Design review of the part built by this model. Coordinates are the model's own, in mm. Face numbers are marked on the shaded views. A direction names the side the tool comes from. Coordinates: 2 decimals unless noted, no trailing zeros. Loops run counter-clockwise (first coordinate to the right, second up) from the corner with the lowest first, then second, coordinate; pieces in that order, holes last. Notation, with made-up numbers: (77, 81.25) - (97, 81.25) arc R28 ccw to (97, 99.25) - close; hole circle Ø1 at (49, -11.75). An arc over 180 degrees is marked (long way). Answer in a Markdown table with one row per item. Add a question column.
(1) To check wall thickness, follow L1, parallel to Y at x = 15.8, z = 35.05; L2, parallel to Y at x = 15, z = 34; L3, parallel to Z at x = -3.5, y = -14. State the ranges of each line that lie inside material, in increasing order. Write a range as [from, to].
(2) Clearance check with flat-ended pins moving along their axes: pin 1 (0.7 mm diameter, centred on y = -0.5, z = 49.5, fed in from -X); pin 2 (2.5 mm diameter, centred on x = -16, y = -15, fed in from +Z); pin 3 (1.5 mm diameter, centred on x = -15.5, y = 15.5, fed in from +Z). State where each tip first meets the part, or that it passes through.
(3) We need section C-C, the plane y = 15.8. Write out the cut boundary in (x, z).
(4) We need section A-A, the plane y = -12.5. Write out the cut boundary in (x, z), plus the area to 3 significant figures.
(5) For the marked faces 1 and 2, list the 3-axis set-ups (+Z, -Z, +X, -X, +Y, -Y) from which the entire face can be reached by the end or side of a thin tool; tool diameter is ignored.
(6) We need section B-B, the plane x = 0. Write out the cut boundary in (y, z), plus the area to 3 significant figures.
(7) The part is to be moulded in two halves that separate along X. For the marked faces 3, 4 and 5, say which applies: released by +X, released by -X, zero draft, split by the parting line, or undercut.
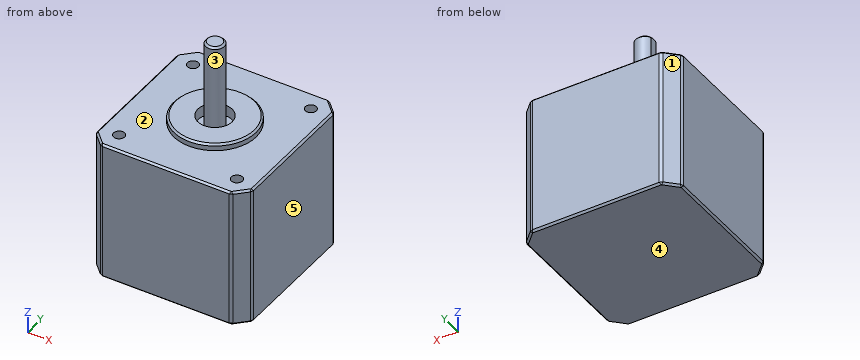
Autodesk Inventor part; units mm, degrees
ref_plane "YZ Plane" through (0, 0, 0) normal (1, 0, 0) x (0, 1, 0)
ref_plane "XZ Plane" through (0, 0, 0) normal (0, 1, 0) x (-1, 0, 0)
ref_plane "XY Plane" through (0, 0, 0) normal (0, 0, 1) x (1, 0, 0)
sketch "Sketch1" plane through (0, 0, 0) normal (0, 0, 1) x (1, 0, 0)
  line L0 (-17.4645, 21) -> (17.4645, 21)
  line L1 (21, 17.4645) -> (21, -17.4645)
  line L2 (17.4645, -21) -> (-17.4645, -21)
  line L3 (-21, -17.4645) -> (-21, 17.4645)
  line L4 (-21, 17.4645) -> (-17.4645, 21)
  line L5 (-21, 17.4645) -> (-16, 17.4645) construction
  line L6 (-17.4645, -21) -> (-21, -17.4645)
  line L7 (21, -17.4645) -> (17.4645, -21)
  line L8 (17.4645, 21) -> (21, 17.4645)
  point P0 (0, 0)
  point P1 (0, 21)
  point P2 (-21, 0)
  dimension "d4" = 360
  dimension "d1" = 45
  dimension "d6" = 5
  dimension "d7" = 42
  dimension "d8" = 42
extrude "Extrusion1" add sketch "Sketch1" along normal blind 37.5
sketch "Sketch2" plane through (0, 0, 37.5) normal (0, 0, 1) x (1, 0, 0)
  circle A0 centre (0, 0) radius 11
  dimension "d11" = 22
extrude "Extrusion2" add sketch "Sketch2" along normal blind 1.8
sketch "Sketch3" plane through (0, 0, 39.3) normal (0, 0, 1) x (1, 0, 0)
  circle A0 centre (0, 0) radius 4.6
  dimension "d14" = 9.2
extrude "Extrusion3" cut sketch "Sketch3" against normal blind 3
sketch "Sketch4" plane through (0, 0, 36.3) normal (0, 0, 1) x (1, 0, 0)
  circle A0 centre (0, 0) radius 2.5
  dimension "d17" = 5
extrude "Extrusion4" add sketch "Sketch4" along normal blind 24
sketch "Sketch5" plane through (0, 0, 60.3) normal (0, 0, 1) x (1, 0, 0)
  arc A0 (-2.25, 1.0897) -> (-2.25, -1.0897) centre (0, 0) ccw
  line L0 (-2.25, 1.0897) -> (-2.25, -1.0897)
  circle A1 centre (0, 0) radius 2.5
  dimension "d20" = 2.25
extrude "Extrusion5" cut sketch "Sketch5" against normal blind 21 contours L0 A0
chamfer "Chamfer1" distance 0.5 angle 45 2 edges at (0.559, -2.4367, 60.3) (0.559, 2.4367, 60.3)
sketch "Sketch6" plane through (0, 0, 37.5) normal (0, 0, 1) x (1, 0, 0)
  circle A0 centre (-15.8, 15.8) radius 1.5
  circle A1 centre (15.8, 15.8) radius 1.5
  circle A2 centre (-15.8, -15.8) radius 1.5
  circle A3 centre (15.8, -15.8) radius 1.5
  point P0 (0, 0)
  dimension "d27" = 15.8
  dimension "d28" = 31.6
  dimension "d29" = 15.8
  dimension "d30" = 31.6
  dimension "d31" = 3
extrude "Extrusion6" cut sketch "Sketch6" against normal blind 5
thread "Thread1"
thread "Thread2"
thread "Thread3"
thread "Thread4"
chamfer "Chamfer2" distance 0.5 angle 45 1 edges at (-11, 0, 39.3)
chamfer "Chamfer3" distance 0.5 angle 45 24 edges at (0, -21, 0) (19.2322, -19.2322, 0) (21, 0, 0) (-21, 0, 0) (0, 21, 0) (21, 0, 37.5) (0, 21, 37.5) (-21, 0, 37.5) (0, -21, 37.5) (19.2322, 19.2322, 37.5) (-19.2322, -19.2322, 37.5) (19.2322, -19.2322, 37.5) (17.4645, -21, 18.75) (21, -17.4645, 18.75) (-17.4645, -21, 18.75) (-21, -17.4645, 18.75) (21, 17.4645, 18.75) (17.4645, 21, 18.75) (-17.4645, 21, 18.75) (-21, 17.4645, 18.75) (-19.2322, 19.2322, 0) (-19.2322, -19.2322, 0) (19.2322, 19.2322, 0) (-19.2322, 19.2322, 37.5)
equation "\"d30\" = d28"
properties part number "Stepper Motor"
Responses:
| question | item | result |
|---|---|---|
| 1 | L1 | y = [-21, -17.3], [-14.3, 14.3], [17.3, 21] |
| 1 | L2 | y = [-21, -17.07], [-14.53, 14.53], [17.07, 21] |
| 1 | L3 | z = [0, 37.5] |
| 2 | pin 1 | stops at x = -2.25 |
| 2 | pin 2 | stops at z = 37.5 |
| 2 | pin 3 | stops at z = 32.5 |
| 3 | outline | (-21, 0.5) - (-20.5, 0) - (20.5, 0) - (21, 0.5) - (21, 37) - (20.5, 37.5) - (17.3, 37.5) - (17.3, 32.5) - (14.3, 32.5) - (14.3, 37.5) - (-14.3, 37.5) - (-14.3, 32.5) - (-17.3, 32.5) - (-17.3, 37.5) - (-20.5, 37.5) - (-21, 37) - close |
| 4 | outline | (-21, 0.5) - (-20.5, 0) - (20.5, 0) - (21, 0.5) - (21, 37) - (20.5, 37.5) - (-20.5, 37.5) - (-21, 37) - close |
| 4 | area | 1,570 mm2 |
| 5 | face 1 | +Z, -Z, -X, +Y |
| 5 | face 2 | +Z |
| 6 | outline | (-21, 0.5) - (-20.5, 0) - (20.5, 0) - (21, 0.5) - (21, 37) - (20.5, 37.5) - (11, 37.5) - (11, 38.8) - (10.5, 39.3) - (4.6, 39.3) - (4.6, 36.3) - (2.5, 36.3) - (2.5, 59.8) - (2, 60.3) - (-2, 60.3) - (-2.5, 59.8) - (-2.5, 36.3) - (-4.6, 36.3) - (-4.6, 39.3) - (-10.5, 39.3) - (-11, 38.8) - (-11, 37.5) - (-20.5, 37.5) - (-21, 37) - close |
| 6 | area | 1,710 mm2 |
| 7 | face 3 | undercut |
| 7 | face 4 | zero draft |
| 7 | face 5 | released by +X |
